Check sheet for the modelled part. Datum: model origin and axes. Units: mm. A direction names the side the tool comes from. Coordinates: 2 decimals unless noted, no trailing zeros. Loops run counter-clockwise (first coordinate to the right, second up) from the corner with the lowest first, then second, coordinate; pieces in that order, holes last.
Autodesk Inventor part; units mm, degrees
ref_plane "YZ Plane" through (0, 0, 0) normal (1, 0, 0) x (0, 1, 0)
ref_plane "XZ Plane" through (0, 0, 0) normal (0, 1, 0) x (-1, 0, 0)
ref_plane "XY Plane" through (0, 0, 0) normal (0, 0, 1) x (1, 0, 0)
sketch "Szkic1" plane through (0, 0, 0) normal (0, 0, 1) x (1, 0, 0)
  line L0 (-11.2555, 18.1319) -> (4.4445, 18.1319)
  line L1 (4.4445, 18.1319) -> (4.4445, -3.8681)
  line L2 (4.4445, -3.8681) -> (-11.2555, -3.8681)
  line L3 (-11.2555, -3.8681) -> (-11.2555, 18.1319)
  line L4 (-11.2555, 2.6319) -> (4.4445, 2.6319)
  line L5 (-11.2555, 11.6319) -> (4.4445, 11.6319)
  point P0 (0, 0)
  dimension "d0" = 15.7
  dimension "d1" = 22
  dimension "d2" = 9
  dimension "d3" = 6.5
  dimension "d4" = 6.5
extrude "Wyciągnięcie proste1" add sketch "Szkic1" along normal blind 1.5 contours L0 L1 L5 L3 | L4 L1 L2 L3
sketch "Szkic2" plane through (0, 0, 1.5) normal (0, 0, 1) x (1, 0, 0)
  line L0 (-11.2555, 18.1319) -> (-11.2555, 11.6319)
  line L1 (-11.2555, 18.1319) -> (-11.2555, 11.6319)
  line L2 (-11.2555, 11.6319) -> (4.4445, 11.6319)
  line L3 (4.4445, 11.6319) -> (4.4445, 18.1319)
  line L4 (4.4445, 18.1319) -> (-11.2555, 18.1319)
  line L5 (4.4445, -3.8681) -> (4.4445, 2.6319)
  line L6 (4.4445, 2.6319) -> (-11.2555, 2.6319)
  line L7 (-11.2555, 2.6319) -> (-11.2555, -3.8681)
  line L8 (-11.2555, -3.8681) -> (4.4445, -3.8681)
  line L9 (4.4445, 18.1319) -> (-11.2555, 18.1319)
  line L10 (-11.2555, 18.1319) -> (4.4445, 18.1319)
  line L11 (4.4445, 18.1319) -> (4.4445, -3.8681)
  line L12 (4.4445, -3.8681) -> (-11.2555, -3.8681)
  line L13 (-11.2555, -3.8681) -> (-11.2555, 18.1319)
  point P0 (0, 0)
extrude "Wyciągnięcie proste2" add sketch "Szkic2" along normal blind 5
sketch "Szkic3" plane through (0, 0, 6.5) normal (0, 0, 1) x (1, 0, 0)
  line L0 (-11.2555, 11.6319) -> (4.4445, 11.6319)
  line L1 (4.4445, 2.6319) -> (-11.2555, 2.6319)
  line L2 (-11.2555, 18.1319) -> (-11.2555, -3.8681)
  line L3 (-11.2555, -3.8681) -> (4.4445, -3.8681)
  line L4 (4.4445, -3.8681) -> (4.4445, 18.1319)
  line L5 (4.4445, 18.1319) -> (-11.2555, 18.1319)
  point P0 (0, 0)
  point P1 (-7.7555, 13.6319)
  point P2 (0.9445, 13.6319)
  point P3 (-7.7555, 0.6319)
  point P4 (0.9445, 0.6319)
  dimension "d9" = 2
  dimension "d10" = 2
  dimension "d11" = 2
  dimension "d12" = 2
  dimension "d13" = 15.7
  dimension "d14" = 3.5
  dimension "d15" = 3.5
  dimension "d16" = 3.5
  dimension "d17" = 3.5
hole "Otwór1" at (-7.7555, 13.6319, 6.5) at (0.9445, 13.6319, 6.5) at (-7.7555, 0.6319, 6.5) at (0.9445, 0.6319, 6.5) direction (0, 0, -1) diameter 3 end through all
sketch "Szkic5" plane through (-11.2555, 2.6319, 0) normal (0, 1, 0) x (1, 0, 0)
  line L0 (0, 0) -> (15.7, 0)
  line L1 (15.7, 0) -> (15.7, -6.5)
  line L2 (0, -6.5) -> (15.7, -6.5)
  line L3 (0, 0) -> (0, -6.5)
  line L4 (12.8, -0.5) -> (12, -0.5)
  line L5 (12, -0.5) -> (12, -1.5)
  line L6 (10.8, -0.5) -> (10.8, -1.5)
  line L7 (10.8, -0.5) -> (10, -0.5)
  line L8 (10, -0.5) -> (10, -1.5)
  line L9 (8.8, -0.5) -> (8.8, -1.5)
  line L10 (8.8, -0.5) -> (8, -0.5)
  line L11 (8, -0.5) -> (8, -1.5)
  line L12 (6.8, -0.5) -> (6.8, -1.5)
  line L13 (6.8, -0.5) -> (6, -0.5)
  line L14 (6, -0.5) -> (6, -1.5)
  line L15 (4.8, -0.5) -> (4.8, -1.5)
  line L16 (4.8, -0.5) -> (4, -0.5)
  line L17 (4, -0.5) -> (4, -1.5)
  line L18 (2.8, -0.5) -> (2.8, -1.5)
  line L19 (2.8, -0.5) -> (2, -0.5)
  line L20 (2, -0.5) -> (2, -1.5)
  line L21 (0.8, -0.5) -> (0.8, -1.5)
  line L22 (0.8, -0.5) -> (0, -0.5)
  line L23 (12.8, -0.5) -> (12.8, -1.5)
  line L24 (14, -1.5) -> (14, -0.5)
  line L25 (14, -0.5) -> (14.8, -0.5)
  line L26 (14.8, -0.5) -> (14.8, -1.5)
  line L27 (0, -1.5) -> (0.8, -1.5)
  line L28 (2, -1.5) -> (2.8, -1.5)
  line L29 (4, -1.5) -> (4.8, -1.5)
  line L30 (6, -1.5) -> (6.8, -1.5)
  line L31 (8, -1.5) -> (8.8, -1.5)
  line L32 (10, -1.5) -> (10.8, -1.5)
  line L33 (12, -1.5) -> (12.8, -1.5)
  line L34 (14, -1.5) -> (14.8, -1.5)
  line L35 (0, -1.5) -> (0, -0.5)
  line L36 (0, 0) -> (0, -6.5)
  point P0 (11.2555, 0)
  dimension "d27" = 0.8
  dimension "d28" = 1.2
  dimension "d41" = 1
  dimension "d42" = 0.5
  dimension "d43" = 0.5
  dimension "d44" = 0.5
  dimension "d45" = 0.5
  dimension "d46" = 0.5
  dimension "d47" = 0.5
  dimension "d48" = 0.5
  dimension "d49" = 0.5
  dimension "d50" = 1
extrude "Wyciągnięcie proste3" add sketch "Szkic5" along normal blind 9 contours L22 L21 L27 L3 | L23 L33 L5 L4 | L6 L32 L8 L7 | L9 L31 L11 L10 | L12 L30 L14 L13 | L15 L29 L17 L16 | L18 L28 L20 L19 | L24 L25 L26 L34
fillet "Zaokrąglenie1" radius 0.2 16 edges at (-9.2555, 7.1319, 0.5) (-8.4555, 7.1319, 0.5) (-7.2555, 7.1319, 0.5) (-6.4555, 7.1319, 0.5) (-5.2555, 7.1319, 0.5) (-4.4555, 7.1319, 0.5) (-3.2555, 7.1319, 0.5) (-2.4555, 7.1319, 0.5) (-1.2555, 7.1319, 0.5) (-0.4555, 7.1319, 0.5) (0.7445, 7.1319, 0.5) (1.5445, 7.1319, 0.5) (2.7445, 7.1319, 0.5) (3.5445, 7.1319, 0.5) (-10.4555, 7.1319, 0.5) (-11.2555, 7.1319, 0.5)
chamfer "Faza1" distance 0.5 angle 45 4 edges at (-11.2555, -3.8681, 3.25) (4.4445, -3.8681, 3.25) (-11.2555, 18.1319, 3.25) (4.4445, 18.1319, 3.25)
equation "\"d43\" = d42"
equation "\"d44\" = d42"
equation "\"d45\" = d42"
equation "\"d46\" = d42"
equation "\"d47\" = d42"
equation "\"d48\" = d42"
equation "\"d49\" = d42"
properties part number "3DP_ABS_X_Axis_Timing_Belt_Clamp"
1) Mould release check, pull along Y, two halves, no side actions. Record for faces 4 (the flat face through (-4, 18.132, 3)), 5 (the flat face through (-4, -3.868, 3)), 6 (the flat face through (-10, 7, 1.5)): +Y half, -Y half, draft (parallel to the pull), parting line (faces both ways), or undercut.
Answer sheet:
face 4: +Y half
face 5: -Y half
face 6: undercut
2) Scan lines: line 1 (X direction, y = 2, z = 0.5); line 2 (Y direction, x = -2.25, z = 1); line 3 (Y direction, x = 1.5, z = 4.5). Record each from-to range of solid material in increasing order.
Answer sheet:
line 1: x = -11.26 to -8.37, -7.14 to 0.33, 1.56 to 4.44
line 2: y = -3.87 to 2.63, 11.63 to 18.13
line 3: y = -3.87 to -0.76, 2.03 to 12.24, 15.03 to 18.13
3) Section check A-A on z = 2.5. Enter the section's corners in (x, y), plus the area to 3 significant figures.
Answer sheet:
outline: (-11.26, -3.37) - (-10.76, -3.87) - (3.94, -3.87) - (4.44, -3.37) - (4.44, 17.63) - (3.94, 18.13) - (-10.76, 18.13) - (-11.26, 17.63) - close; hole circle Ø3 at (-7.76, 0.63); hole circle Ø3 at (-7.76, 13.63); hole circle Ø3 at (0.94, 0.63); hole circle Ø3 at (0.94, 13.63)
area: 317 mm2
4) Section check B-B on x = -4. Enter the section's corners in (y, z), plus the area to 4 significant figures.
Answer sheet:
outline: (-3.87, 0) - (2.63, 0) - (2.63, 1.5) - (11.63, 1.5) - (11.63, 0) - (18.13, 0) - (18.13, 6.5) - (-3.87, 6.5) - close
area: 129.5 mm2
5) Set-up check for faces 1 (the flat face through (2, 7, 1.5)), 2 (the cylindrical face through (1.86, 1.82, 3.2)), 3 (the flat face through (4, 7, 1.5)): record each of +Z, -Z, +X, -X, +Y, -Y from which the full face is reachable in a straight line by a thin tool's end or side.
Answer sheet:
face 1: -Z
face 2: +Z, -Z
face 3: -Z, +X
6) Depth check by flat-ended pin: pin 1 (0.9 mm diameter, centred on y = 6, z = 1, fed in from +X); pin 2 (0.6 mm diameter, centred on x = -10, y = 7.5, fed in from -Z); pin 3 (1.3 mm diameter, centred on x = -2, y = 6.5, fed in from -Z). Enter the tip coordinate at first touch or a pass-through.
Answer sheet:
pin 1: stops at x = 3.54
pin 2: stops at z = 1.5
pin 3: stops at z = 0.5
7) Section check C-C on z = 1. Give the number of separate pieces and of enclosed holes in the cut face, plus the area to 3 significant figures.
Answer sheet:
separate pieces: 1
enclosed holes: 11
area: 233 mm2
